from build123d import *

# Parameters (mm, degrees)
PAD_DEPTH = 10
FILLET_R  = 0.8


with BuildPart() as part:
    # Sketch → Pad (new body)
    with BuildSketch(Plane.XY):
        Polygon((-4, 4.8), (-4, -4.8), (4, -4.8), (4, 4.8), (1.2, 4.8), (1.2, -2), (-1.2, -2), (-1.2, 4.8), align=None)
    extrude(amount=PAD_DEPTH)

    # Fillet
    fillet_edges = [part.edges().sort_by_distance(p)[0] for p in [
        (-4, -4.8, 5),
        (4, -4.8, 5),
        (4, 4.8, 5),
        (1.2, 4.8, 5),
        (-4, 4.8, 5),
        (-1.2, 4.8, 5),
    ]]
    fillet(fillet_edges, radius=FILLET_R)


solid = part.part
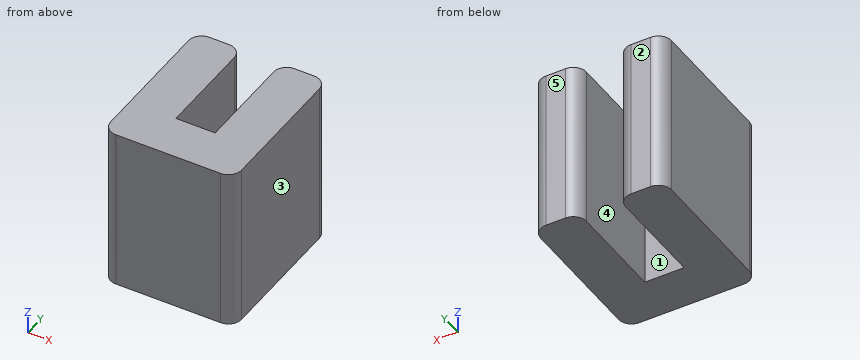
The model under review builds one solid part; all positions refer to its coordinate system, in mm. Face numbers are marked on the shaded views. A direction names the side the tool comes from. Round coordinates to 2 decimals unless told otherwise and drop trailing zeros. Write each loop counter-clockwise with the first axis right and the second up, starting at its lowest first coordinate (ties: lowest second). Pieces come first, ordered by that corner, then holes. Notation, with made-up numbers: (52, 20) - (96, 20) arc R31 cw to (96, 46) - close; hole circle Ø4 at (-39.75, -6.75). An arc over 180 degrees is marked (long way). One line per item, written item: value. Start each with the question number.
1. Machinability: for the marked faces 4 and 5, which of the approach directions +Z, -Z, +X, -X, +Y, -Y give a long, thin tool a straight path to every point of the face, cutting with its end or side? Answer none if there is none.
2. To check wall thickness, follow L1, parallel to X at y = 1.25, z = 3.5; L2, parallel to Y at x = 1, z = 6.75; L3, parallel to Y at x = -3.5, z = 4.5. State the ranges of each line that lie inside material, in increasing order. Write a range as from..to.
3. Consider section C-C on x = -1. Write out the cut boundary in (y, z).
4. Clearance check with flat-ended pins moving along their axes: P1, Ø4, axis at x = -1, y = -2.5, coming from the -Z side; P2, Ø1.2, axis at x = 0, z = 6.5, coming from the +Y side. State where each tip first meets the part, or that it passes through.
5. Consider section A-A on y = 2.25. Write out the cut boundary in (x, z).
6. Consider section B-B on z = 2.25. Write out the cut boundary in (x, y).
7. The part is to be moulded in two halves that separate along X. For the marked faces 1, 2 and 3, say which applies: released by +X, released by -X, zero draft, split by the parting line, or undercut.
Checks:
1. face 4: +Z, -Z, +Y
1. face 5: +Z, -Z, +X, -X, +Y
2. L1: x = -4..-1.2, 1.2..4
2. L2: y = -4.8..-2
2. L3: y = -4.74..4.74
3. outline: (-4.8, 0) - (-2, 0) - (-2, 10) - (-4.8, 10) - close
4. P1: stops at z = 0
4. P2: stops at y = -2
5. outline: (-4, 0) - (-1.2, 0) - (-1.2, 10) - (-4, 10) - close; (1.2, 0) - (4, 0) - (4, 10) - (1.2, 10) - close
6. outline: (-4, -4) arc R0.8 ccw to (-3.2, -4.8) - (3.2, -4.8) arc R0.8 ccw to (4, -4) - (4, 4) arc R0.8 ccw to (3.2, 4.8) - (2, 4.8) arc R0.8 ccw to (1.2, 4) - (1.2, -2) - (-1.2, -2) - (-1.2, 4) arc R0.8 ccw to (-2, 4.8) - (-3.2, 4.8) arc R0.8 ccw to (-4, 4) - close
7. face 1: undercut
7. face 2: zero draft
7. face 3: released by +X
